Can you work these out from the model? Positions are in its coordinate system, mm. Face numbers are marked on the shaded views. A direction names the side the tool comes from. Coordinates: 2 decimals unless noted, no trailing zeros. Loops run counter-clockwise (first coordinate to the right, second up) from the corner with the lowest first, then second, coordinate; pieces in that order, holes last. Notation, with made-up numbers: (-23.75, 25.5) -> (23.25, 25.5) arc R29 cw to (23.25, 61.5) -> close; hole circle Ø3 at (-6.5, 62). An arc over 180 degrees is marked (long way). Use one line per item in the form item = value. Start each with the question number.
(1) On a 3-axis mill with a long thin cutter (end or side, diameter ignored), from which of +Z, -Z, +X, -X, +Y, -Y can I reach the whole of each face in a straight line? I mean the marked faces 4, 5 and 6. Say none if no direction works.
(2) Imagine slicing it at D-D (z = 80). State how many separate pieces and enclosed holes the cut face has, plus the area to 3 significant figures.
(3) Thinking about a two-plate mould opening in Y: for the marked faces 1, 2 and 3, which applies, released by +Y, released by -Y, zero draft, split by the parting line, or undercut?
(4) Imagine slicing it at A-A (x = 42.5). List the corners of the cut face in (y, z) for me (3 decimals), plus the area to 3 significant figures.
(5) Imagine slicing it at B-B (z = 58.5). List the corners of the cut face in (x, y) for me, plus the area to 3 significant figures.
(6) Imagine slicing it at C-C (y = -51.5). List the corners of the cut face in (x, z) for me, plus the area to 3 significant figures.
(7) I'm going to push flat-ended pins straight in: pin 1 (7.5 mm diameter, centred on x = 61.5, z = 78, fed in from +Y); pin 2 (7 mm diameter, centred on y = 0, z = 58.5, fed in from +X); pin 3 (13 mm diameter, centred on y = 0.5, z = -59.5, fed in from +X); pin 4 (3.5 mm diameter, centred on y = 0, z = 58.5, fed in from +X). Where does each tip first touch, or does it pass through?
(8) I need wall thicknesses on line 1 (Z direction, x = 24.5, y = -52); line 2 (Z direction, x = 45, y = -84.5) (3 decimals); line 3 (Z direction, x = 24, y = -87). Which ranges of each line are inside material? Lowest first, please. Write a range as [from, to].
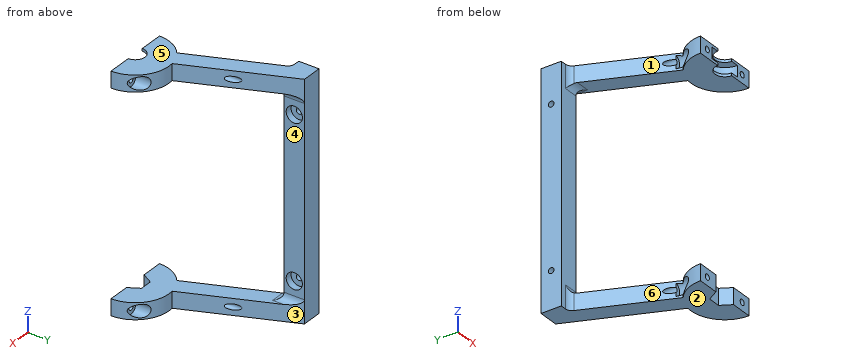
```python
from build123d import *

# Parameters (mm, degrees)
SKETCH1_W               = 15
SKETCH1_H               = 15
BOSS_EXTRUDE1_DEPTH     = 86
BOSS_EXTRUDE2_DEPTH     = 12
SKETCH3_R               = 6
CUT_EXTRUDE1_DEPTH      = 5
SKETCH4_R               = 2.1
CUT_EXTRUDE2_DEPTH      = 135.726016512
BOSS_EXTRUDE5_DEPTH     = 12
SKETCH8_R               = 4.75
CUT_EXTRUDE4_DEPTH      = 4
CUT_EXTRUDE4_DEPTH_BACK = 10
SKETCH6_R               = 2.1
CUT_EXTRUDE5_DEPTH      = 149.162917192
FILLET1_R               = 5
CUT_EXTRUDE6_REACH      = 208.631
SKETCH9_R               = 7.2
CUT_EXTRUDE7_START      = -1.925
SKETCH10_R              = 13.1
CUT_EXTRUDE7_DEPTH      = 8.15
CUT_EXTRUDE8_REACH      = 208.631


with BuildPart() as part:
    # Sketch1 → Boss-Extrude1 (new body)
    with BuildSketch(Plane.XY):
        Rectangle(SKETCH1_W, SKETCH1_H)
    extrude(amount=BOSS_EXTRUDE1_DEPTH)

    # Sketch2 → Boss-Extrude2 (add)
    with BuildSketch(Plane.XY.offset(86)):
        Polygon((7.5, 7.5), (49.391891892, -92.5), (35.608108108, -92.5), (0, -7.5), align=None)
    extrude(amount=-BOSS_EXTRUDE2_DEPTH)

    # Sketch3 → Cut-Extrude1 (cut)
    with BuildSketch(Plane(origin=(7.5, 0, 0), x_dir=(0, 0, -1), z_dir=(1, 0, 0))):
        with Locations((-58.5, 0)):
            Circle(SKETCH3_R)
    extrude(amount=-CUT_EXTRUDE1_DEPTH, mode=Mode.SUBTRACT)

    # Sketch4 → Cut-Extrude2 (cut, through all)
    with BuildSketch(Plane(origin=(2.5, 0, 0), x_dir=(0, 0, -1), z_dir=(1, 0, 0))):
        with Locations((-58.5, 0)):
            Circle(SKETCH4_R)
    extrude(amount=-CUT_EXTRUDE2_DEPTH, mode=Mode.SUBTRACT)

    # Sketch5 → Boss-Extrude5 (add)
    with BuildSketch(Plane.XY.offset(86)):
        with BuildLine():
            Line((17.5, -92.5), (67.5, -92.5))
            ThreePointArc((67.5, -92.5), (42.5, -67.5), (17.5, -92.5))
        make_face()
    extrude(amount=-BOSS_EXTRUDE5_DEPTH)

    # Sketch8 → Cut-Extrude4 (cut, two sides)
    with BuildSketch(Plane(origin=(0, -72.655502084, 0), x_dir=(1, 0, 0), z_dir=(0, 1, 0))) as cut_extrude4_sk:
        with Locations(Location((24.5, -80, 0), (0, 0, 76.371804965))):
            Circle(SKETCH8_R)
        with Locations(Location((60.5, -80, 0), (0, 0, 90))):
            Circle(SKETCH8_R)
    extrude(amount=CUT_EXTRUDE4_DEPTH, mode=Mode.SUBTRACT)
    extrude(cut_extrude4_sk.sketch, amount=-CUT_EXTRUDE4_DEPTH_BACK, mode=Mode.SUBTRACT)

    # Sketch6 → Cut-Extrude5 (cut, through all)
    with BuildSketch(Plane.XZ.offset(92.5)):
        with Locations(Location((24.5, 80, 0), (0, 0, 270))):
            Circle(SKETCH6_R)
        with Locations(Location((60.5, 80, 0), (0, 0, 90))):
            Circle(SKETCH6_R)
    extrude(amount=-CUT_EXTRUDE5_DEPTH, mode=Mode.SUBTRACT)

    # Fillet1
    fillet1_edges = [part.edges().sort_by_distance(p)[0] for p in [
        (3.75, -7.5, 74),
        (7.5, 0, 74),
        (0, -7.5, 80),
    ]]
    fillet(fillet1_edges, radius=FILLET1_R)

    # Mirror2: part across plane


with BuildPart() as part_1:
    add(part.part)
    add(part.part.mirror(Plane(origin=(0, 0, 0), x_dir=(1, 0, 0), z_dir=(0, 0, -1))))

    # Sketch9 → Cut-Extrude6 (cut, up to next)
    with BuildSketch(Plane.XY.offset(86), mode=Mode.PRIVATE) as cut_extrude6_sk1:
        with Locations((42.5, -92.5)):
            Circle(SKETCH9_R)
    cut_extrude6_tool1 = extrude(cut_extrude6_sk1.sketch, amount=-CUT_EXTRUDE6_REACH, mode=Mode.PRIVATE) & part_1.part
    add(cut_extrude6_tool1.solids().sort_by_distance((42.5, -92.5, 86))[0], mode=Mode.SUBTRACT)

    # Sketch10 → Cut-Extrude7 (cut)
    with BuildSketch(Plane.XY.offset(86).offset(CUT_EXTRUDE7_START)):
        with Locations((42.5, -92.5)):
            Circle(SKETCH10_R)
    extrude(amount=-CUT_EXTRUDE7_DEPTH, mode=Mode.SUBTRACT)

    # Sketch11 → Cut-Extrude8 (cut, up to next)
    with BuildSketch(Plane(origin=(0, 0, -86), x_dir=(-1, 0, 0), z_dir=(0, 0, -1)), mode=Mode.PRIVATE) as cut_extrude8_sk1:
        Polygon((-33.4, -92.5), (-37.95, -84.619168826), (-47.05, -84.619168826), (-51.6, -92.5), (-47.05, -100.380831174), (-37.95, -100.380831174), align=None)
    cut_extrude8_tool1 = extrude(cut_extrude8_sk1.sketch, amount=-CUT_EXTRUDE8_REACH, mode=Mode.PRIVATE) & part_1.part
    add(cut_extrude8_tool1.solids().sort_by_distance((42.5, -92.5, -86))[0], mode=Mode.SUBTRACT)


solid = part_1.part
```
Worked out:
q1.face_4 = +X, +Y, -Y
q1.face_5 = +Z, +X, -X, +Y, -Y
q1.face_6 = +Z, -Z, -X
q2.separate_pieces = 4
q2.enclosed_holes = 0
q2.area = 1,480 mm2
q3.face_1 = undercut
q3.face_2 = zero draft
q3.face_3 = released by +Y
q4.outline = (-85.3, 74) -> (-67.5, 74) -> (-67.5, 86) -> (-85.3, 86) -> (-85.3, 84.075) -> (-79.4, 84.075) -> (-79.4, 75.925) -> (-85.3, 75.925) -> close; (-84.619, -86) -> (-67.5, -86) -> (-67.5, -74) -> (-84.619, -74) -> close
q4.area = 371 mm2
q5.outline = (-7.5, -7.5) -> (7.5, -7.5) -> (7.5, -6) -> (2.5, -6) -> (2.5, -2.1) -> (-7.5, -2.1) -> close; (-7.5, 2.1) -> (2.5, 2.1) -> (2.5, 6) -> (7.5, 6) -> (7.5, 7.5) -> (-7.5, 7.5) -> close
q5.area = 123 mm2
q6.outline = (18.43, -86) -> (32.22, -86) -> (32.22, -74) -> (18.43, -74) -> close; (18.43, 74) -> (32.22, 74) -> (32.22, 86) -> (18.43, 86) -> close; hole circle Ø4.2 at (24.5, -80); hole circle Ø4.2 at (24.5, 80)
q6.area = 303 mm2
q7.pin_1 = -73.35
q7.pin_2 = 2.5
q7.pin_3 = 7.5
q7.pin_4 = through
q8.line_1 = [-86, -82.1], [-77.9, -74], [74, 77.9], [82.1, 86]
q8.line_2 = [-86, -74], [74, 75.925], [84.075, 86]
q8.line_3 = [-86, -82.04], [-77.96, -74], [74, 77.96], [82.04, 86]
